```python
from build123d import *

# Parameters (mm, degrees)
BASE_FLANGE1_DEPTH = 6.35
FILLET1_R          = 3.175
FILLET2_R          = 0.79375


# Sheet-metal steps are written as plain solids
with BuildPart() as part:
    # Sketch1 → Base-Flange1 (new body)
    with BuildSketch(Plane(origin=(0, 0, 0), x_dir=(0, 0, -1), z_dir=(1, 0, 0))):
        Polygon((-56.35625, 0), (-12.7, 50.8), (25.4, 50.8), (25.4, 38.1), (0, 38.1), (0, 0), (-13.096875, 0), (-13.096875, -12.7), (-37.703125, -12.7), (-37.703125, 0), align=None)
    extrude(amount=-BASE_FLANGE1_DEPTH)

    # Fillet1
    fillet1_edges = [part.edges().sort_by_distance(p)[0] for p in [
        (-3.175, 0, 56.35625),
        (-3.175, 50.8, 12.7),
        (-3.175, 50.8, -25.4),
        (-3.175, 38.1, -25.4),
        (-3.175, 38.1, 0),
        (-3.175, 0, 0),
    ]]
    fillet(fillet1_edges, radius=FILLET1_R)

    # Fillet2
    fillet2_edges = [part.edges().sort_by_distance(p)[0] for p in [
        (-3.175, 0, 13.096875),
        (-3.175, -12.7, 13.096875),
        (-3.175, -12.7, 37.703125),
        (-3.175, 0, 37.703125),
    ]]
    fillet(fillet2_edges, radius=FILLET2_R)


solid = part.part
```
For this review, take the finished solid that the model builds, in its own axes (mm). A direction names the side the tool comes from. Round coordinates to 2 decimals unless told otherwise and drop trailing zeros. Loops run counter-clockwise (first coordinate to the right, second up) from the corner with the lowest first, then second, coordinate; pieces in that order, holes last.
Q1. Insertion check: pin 1 Ø3 at (x, y) = (-0.5, 13.5) entering from -Z; pin 2 Ø3 at (x, z) = (-3, 7.5) entering from -Y; pin 3 Ø3 at (x, y) = (-4, -7) entering from +Z. Each pin has a flat end and moves straight along its axis. Give the tip position at first contact, or say it passes through.
Result sheet:
pin 1: stops at z = 0
pin 2: stops at y = 0
pin 3: stops at z = 37.7
Q2. Machinability: for faces 1 (the face through (-6.35, 19, 13)), 2 (the face through (-3, 0, 44)), 3 (the face through (-3, 38.1, -13)), which of the approach directions +Z, -Z, +X, -X, +Y, -Y give a long, thin tool a straight path to every point of the face, cutting with its end or side? Answer none if there is none.
Result sheet:
face 1: +Z, -Z, -X, +Y, -Y
face 2: +Z, +X, -X, -Y
face 3: -Z, +X, -X, -Y
Q3. Add section C-C on y = -9. Write out the cut boundary in (x, z).
Result sheet:
outline: (-6.35, 13.1) - (0, 13.1) - (0, 37.7) - (-6.35, 37.7) - close
Q4. To check wall thickness, follow line 1 along Y through (x, z) = (-2, -9.5); line 2 along Z through (x, y) = (-3.75, -3.5); line 3 along Z through (x, y) = (-5.5, 44). State the ranges of each line that lie inside material, in increasing order.
Result sheet:
line 1: y = 38.1 to 50.8
line 2: z = 13.1 to 37.7
line 3: z = -25.4 to 18.54
Q5. Add section B-B on z = -20. Write out the cut boundary in (x, y), plus the area to 3 significant figures.
Result sheet:
outline: (-6.35, 38.1) - (0, 38.1) - (0, 50.8) - (-6.35, 50.8) - close
area: 80.6 mm2
